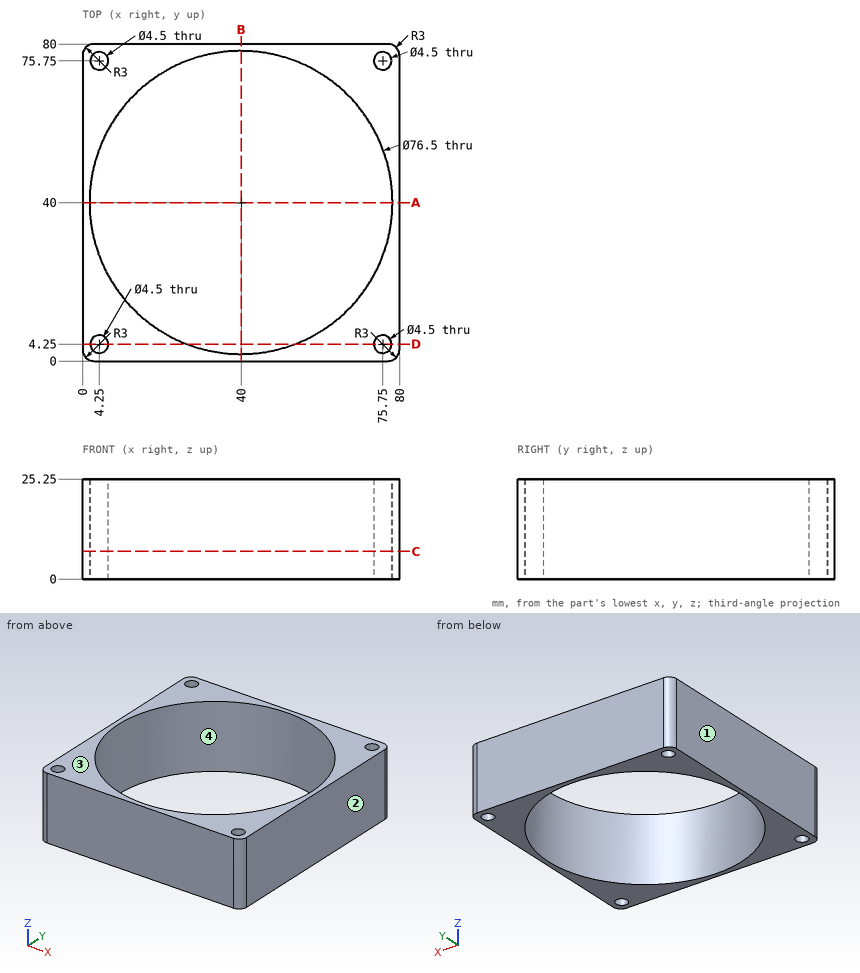
Answer from the drawing. Dimensions are ordinates in mm from the lowest x, y and z of the part. Give positions to 0.01 mm unless a question says otherwise; leave off trailing zeros. Write each loop counter-clockwise with the first axis right and the second up, starting at its lowest first coordinate (ties: lowest second). Pieces come first, ordered by that corner, then holes.
1) Section D-D (y = 4.25) is taken. Write down the section's boundary in (x, z), and give its area (3 significant figures).
2) Section C-C (z = 7) is taken. Write down the section's boundary in (x, y), and give its area (3 significant figures).
3) Find the intervals of material crossed by L1, parallel to Y at x = 40, z = 10.5; L2, parallel to Y at x = 74.5, z = 5.75; L3, parallel to X at y = 35, z = 22.25, in increasing order.
4) Section A-A (y = 40) is taken. Write down the section's boundary in (x, z), and give its area (3 significant figures).
5) Given P1, Ø7, axis at x = 4.25, y = 75.75, coming from the +Z side, flat-ended and moving along its own axis, determine where the tip first touches the part or whether it passes through.
6) For a pull along X with two mould halves and no side action, classify the marked faces 1, 2, 3 and 4 as pulls with the +X half, pulls with the -X half, needs draft (parallel to the pull), parting line crosses it, or undercut.
Response:
1. outline: (0, 0) - (2, 0) - (2, 25.25) - (0, 25.25) - close; (6.5, 0) - (26.4, 0) - (26.4, 25.25) - (6.5, 25.25) - close; (53.6, 0) - (73.5, 0) - (73.5, 25.25) - (53.6, 25.25) - close; (78, 0) - (80, 0) - (80, 25.25) - (78, 25.25) - close
1. area: 1,110 mm2
2. outline: (0, 3) arc R3 ccw to (3, 0) - (77, 0) arc R3 ccw to (80, 3) - (80, 77) arc R3 ccw to (77, 80) - (3, 80) arc R3 ccw to (0, 77) - close; hole circle Ø76.5 at (40, 40); hole circle Ø4.5 at (4.25, 4.25); hole circle Ø4.5 at (4.25, 75.75); hole circle Ø4.5 at (75.75, 4.25); hole circle Ø4.5 at (75.75, 75.75)
2. area: 1,730 mm2
3. L1: y = 0 to 1.75, 78.25 to 80
3. L2: y = 0 to 2.38, 6.12 to 23.48, 56.52 to 73.88, 77.62 to 80
3. L3: x = 0 to 2.08, 77.92 to 80
4. outline: (0, 0) - (1.75, 0) - (1.75, 25.25) - (0, 25.25) - close; (78.25, 0) - (80, 0) - (80, 25.25) - (78.25, 25.25) - close
4. area: 88.4 mm2
5. P1: stops at z = 25.25
6. face 1: pulls with the -X half
6. face 2: pulls with the +X half
6. face 3: needs draft
6. face 4: undercut
